CAD build for the part. Positions are in the model's coordinates, mm. A direction names the side the tool comes from. Give positions to 0.01 mm unless a question says otherwise; leave off trailing zeros. Write each loop counter-clockwise with the first axis right and the second up, starting at its lowest first coordinate (ties: lowest second). Pieces come first, ordered by that corner, then holes. Notation, with made-up numbers: (15.25, -33) - (64.25, -33) arc R35 cw to (64.25, 5) - close; hole circle Ø7 at (1.5, 57.25). An arc over 180 degrees is marked (long way). Put each result on its own line as item: value. Start each with the question number.
1. Tool access for faces 4 (the flat face through (337.031, 472, -698)), 5 (the flat face through (389, 418.098, -694)), 6 (the flat face through (476.461, 444, -698)): list every direction of +Z, -Z, +X, -X, +Y, -Y with a clear straight run to the whole face (end or side of a thin tool).
2. Cut at B-B on y = 430. List the corners of the cut face in (x, z).
3. Wall check: line 1 (X direction, y = 415, z = -713); line 2 (X direction, y = 433, z = -674); line 3 (Y direction, x = 417.5, z = -687). Give the ranges that are in metal, low to high.
4. Drop flat-ended pins along their axis: pin 1 (14 mm diameter, centred on x = 318.5, z = -693, fed in from +Y); pin 2 (5 mm diameter, centred on x = 314.5, z = -685.5, fed in from -Y); pin 3 (3 mm diameter, centred on y = 472, z = -696, fed in from -X). Give the stop position or say it passes through.
5. Cut at C-C on x = 363.5. List the corners of the cut face in (y, z), and give its area (3 significant figures).
6. Mould opens along Y. For faces 1 (the flat face through (408, 477.098, -698)), 2 (the flat face through (380, 476, -670.191)), 3 (the flat face through (315, 461.098, -694)) say: +Y half, -Y half, draft (parallel to the pull), parting line (faces both ways), or undercut.
from build123d import *

# Parameters (mm, degrees)
BOSS_EXTRUDE1_DEPTH     = 4
BOSS_EXTRUDE2_DEPTH     = 50
CUT_EXTRUDE1_DEPTH      = 677.427541211
CUT_EXTRUDE1_DEPTH_BACK = 50
SKETCH3_W               = 22.667747696
SKETCH3_H               = 6
SKETCH3_W_2             = 18
FILLET3_R               = 3


with BuildPart() as part:
    # Sketch1 → Boss-Extrude1 (new body)
    with BuildSketch(Plane.XY.offset(-724.191392871)):
        Polygon((476.461364297, 467.098298929), (476.461364297, 412.098298929), (285.063110998, 412.098298929), (285.063110998, 467.098298929), (337.030633325, 467.098298929), (337.030633325, 477.098298929), (476.461364297, 477.098298929), align=None)
    extrude(amount=BOSS_EXTRUDE1_DEPTH)

    # Sketch2 → Boss-Extrude2 (add)
    with BuildSketch(Plane.XY.offset(-720.191392871)):
        Polygon((285.063110998, 467.098298929), (285.063110998, 412.098298929), (476.461364297, 412.098298929), (476.461364297, 477.098298929), (337.030633325, 477.098298929), (337.030633325, 467.098298929), align=None)
        Polygon((291.063110998, 461.098298929), (343.030633325, 461.098298929), (343.030633325, 471.098298929), (470.461364297, 471.098298929), (470.461364297, 418.098298929), (291.063110998, 418.098298929), align=None, mode=Mode.SUBTRACT)
    extrude(amount=BOSS_EXTRUDE2_DEPTH)

    # Sketch3 → Cut-Extrude1 (cut, two sides: drawn at the far end of the back side and taken through both)
    with BuildSketch(Plane.XY.offset(-670.191392871).offset(-CUT_EXTRUDE1_DEPTH_BACK)):
        with Locations((319.72923715, 415.098298929)):
            Rectangle(SKETCH3_W, SKETCH3_H)
        with Locations((453.461364297, 415.098298929)):
            Rectangle(SKETCH3_W_2, SKETCH3_H)
    extrude(amount=CUT_EXTRUDE1_DEPTH + CUT_EXTRUDE1_DEPTH_BACK, mode=Mode.SUBTRACT)

    # Fillet3
    fillet3_edges = [part.edges().sort_by_distance(p)[0] for p in [
        (337.030633325, 477.098298929, -697.191392871),
        (476.461364297, 477.098298929, -697.191392871),
        (476.461364297, 412.098298929, -697.191392871),
        (285.063110998, 412.098298929, -697.191392871),
        (285.063110998, 467.098298929, -697.191392871),
        (337.030633325, 467.098298929, -697.191392871),
        (343.030633325, 461.098298929, -695.191392871),
        (406.745998811, 471.098298929, -720.191392871),
        (343.030633325, 466.098298929, -720.191392871),
        (317.046872162, 461.098298929, -720.191392871),
        (299.72923715, 418.098298929, -720.191392871),
        (470.461364297, 444.598298929, -720.191392871),
        (387.762237648, 418.098298929, -720.191392871),
        (466.461364297, 418.098298929, -720.191392871),
        (308.395363302, 415.098298929, -670.191392871),
        (331.063110998, 418.098298929, -695.191392871),
        (331.063110998, 415.098298929, -720.191392871),
        (331.063110998, 412.098298929, -695.191392871),
        (308.395363302, 412.098298929, -695.191392871),
        (308.395363302, 418.098298929, -695.191392871),
        (319.72923715, 412.098298929, -720.191392871),
        (308.395363302, 415.098298929, -720.191392871),
        (444.461364297, 412.098298929, -695.191392871),
        (444.461364297, 415.098298929, -720.191392871),
        (444.461364297, 418.098298929, -695.191392871),
        (462.461364297, 412.098298929, -695.191392871),
        (462.461364297, 415.098298929, -720.191392871),
        (453.461364297, 412.098298929, -720.191392871),
    ]]
    fillet(fillet3_edges, radius=FILLET3_R - 0.0001)  # a hair under: the kernel refuses the full size


solid = part.part
Report:
1. face 4: +Z, -Z, -X, +Y
1. face 5: +Z
1. face 6: +Z, -Z, +X, +Y, -Y
2. outline: (285.06, -724.19) - (476.46, -724.19) - (476.46, -670.19) - (470.46, -670.19) - (470.46, -717.19) arc R3 cw to (467.46, -720.19) - (291.06, -720.19) - (291.06, -670.19) - (285.06, -670.19) - close
3. line 1: x = 285.06 to 308.39, 331.06 to 444.46, 462.46 to 476.46
3. line 2: x = 285.06 to 291.06, 470.46 to 476.46
3. line 3: y = 412.1 to 418.1, 471.1 to 477.1
4. pin 1: stops at y = 467.1
4. pin 2: stops at y = 461.1
4. pin 3: stops at x = 337.03
5. outline: (412.1, -724.19) - (477.1, -724.19) - (477.1, -670.19) - (471.1, -670.19) - (471.1, -717.19) arc R3 cw to (468.1, -720.19) - (421.1, -720.19) arc R3 cw to (418.1, -717.19) - (418.1, -670.19) - (412.1, -670.19) - close
5. area: 864 mm²
6. face 1: +Y half
6. face 2: draft
6. face 3: undercut
